Autodesk Inventor part; units mm, degrees
ref_plane "YZ Plane" through (0, 0, 0) normal (1, 0, 0) x (0, 1, 0)
ref_plane "XZ Plane" through (0, 0, 0) normal (0, 1, 0) x (-1, 0, 0)
ref_plane "XY Plane" through (0, 0, 0) normal (0, 0, 1) x (1, 0, 0)
sketch "スケッチ1" plane through (0, 0, 0) normal (0, 1, 0) x (-1, 0, 0)
  circle A0 centre (0, 0) radius 7.5
  dimension "d0" = 15
extrude "押し出し1" add sketch "スケッチ1" along normal blind 110
sketch "スケッチ2" plane through (0, 110, 0) normal (0, 1, 0) x (1, 0, 0)
  circle A0 centre (0, 0) radius 6
  circle A1 centre (0, 0) radius 8
  dimension "d3" = 12
extrude "押し出し2" cut sketch "スケッチ2" against normal blind 20
sketch "スケッチ3" plane through (0, 0, 0) normal (0, -1, 0) x (1, 0, 0)
  circle A0 centre (0, 0) radius 6
  dimension "d6" = 12
extrude "押し出し3" add sketch "スケッチ3" along normal blind 20
properties part number "shaft2016"
Work out the finished part from the listing and answer in its coordinate system (mm). A direction names the side the tool comes from. Round coordinates to 2 decimals unless told otherwise and drop trailing zeros. Order: outer loops, then holes, each group sorted by start corner. A loop starts at its lowest first (then second) coordinate and runs counter-clockwise, first axis right, second up. Notation, with made-up numbers: M 12,45 L 41,45 A23 cw 41,68 Z; hole C 73,22.5 d7. An arc over 180 degrees is marked long. Put each result on its own line as item: value. Start each with the question number.
Q1. Straight lines are drawn through the part: L1, parallel to Y at x = -2.75, z = 6.5; L2, parallel to Z at x = 0.5, y = 11.5; L3, parallel to X at y = 19, z = 0.25. For each, find the intervals that lie inside material, in ascending order. Write a range as [from, to].
Q2. Flat-ended cylindrical pins translate along their axes: pin 1 (2 mm diameter, centred on x = 2, y = 42.5, fed in from -Z); pin 2 (5 mm diameter, centred on y = 10, z = -4.5, fed in from +X); pin 3 (6 mm diameter, centred on y = 11, z = -5.5, fed in from -X). Find the tip coordinate at first contact, or state that the pin passes through.
Q3. A tool of negligible diameter and unlimited length cuts with its end or side. For faces 1 (the flat face through (0, -20, 0)), 2 (the flat face through (-2, 0, 6)), 3 (the cylindrical face through (-6, 100, 0)), from which of +Z, -Z, +X, -X, +Y, -Y can it reach the whole face along a straight path? Write none if from no direction.
Q4. Section A-A, the plane z = 0 is taken. Write down the section's boundary in (x, y).
Q5. Section B-B, the plane x = 0 is taken. Write down the section's boundary in (y, z).
Q6. Section C-C, the plane y = -2 is taken. Write down the section's boundary in (x, z).
Findings below:
1. L1: y = [0, 90]
1. L2: z = [-7.48, 7.48]
1. L3: x = [-7.5, 7.5]
2. pin 1: stops at z = -7.43
2. pin 2: stops at x = 7.23
2. pin 3: stops at x = -7.07
3. face 1: +Z, -Z, +X, -X, -Y
3. face 2: -Y
3. face 3: +Y
4. outline: M -7.5,0 L -6,0 L -6,-20 L 6,-20 L 6,0 L 7.5,0 L 7.5,90 L 6,90 L 6,110 L -6,110 L -6,90 L -7.5,90 Z
5. outline: M -20,-6 L 0,-6 L 0,-7.5 L 90,-7.5 L 90,-6 L 110,-6 L 110,6 L 90,6 L 90,7.5 L 0,7.5 L 0,6 L -20,6 Z
6. outline: C 0,0 d12
